```python
from build123d import *

# Parameters (mm, degrees)
F1_DEPTH = 25.4
F3_R     = 6.35
F4_DEPTH = 25.4
F6_DEPTH = 25.4
F7_W     = 12.7
F7_H     = 7.132675
F8_DEPTH = 19.05


with BuildPart() as f1:
    # F0 (on Front) → F1 (new body)
    with BuildSketch(Plane.XZ):
        Polygon((0, 44.45), (0, 0), (57.15, 0), (57.15, 12.7), (12.7, 12.7), (12.7, 44.45), align=None)
    extrude(amount=F1_DEPTH)

    # F3 (on face) → F4 (cut)
    with BuildSketch(Plane.XY.offset(12.7)):
        with Locations((26.631284, -12.7)):
            Circle(F3_R)
        with Locations((45.681284, -12.7)):
            Circle(F3_R)
    extrude(amount=-F4_DEPTH, mode=Mode.SUBTRACT)

    # F5 (on face) → F6 (cut)
    with BuildSketch(Plane.XY.offset(12.7)):
        with BuildLine():
            ThreePointArc((46.05227, 0), (56.65458, -12.572447), (46.362385, -25.4))
            Line((46.362385, -25.4), (57.15, -25.4))
            Line((57.15, -25.4), (57.15, 0))
            Line((57.15, 0), (46.05227, 0))
        make_face()
    extrude(amount=-F6_DEPTH, mode=Mode.SUBTRACT)

    # F7 (on face) → F8 (cut)
    with BuildSketch(Plane.XY.offset(44.45)):
        with Locations((6.35, -11.474303)):
            Rectangle(F7_W, F7_H)
    extrude(amount=-F8_DEPTH, mode=Mode.SUBTRACT)


solid = f1.part
```
Input: part model. Units: mm. Frame: model coordinates. A direction names the side the tool comes from. Round coordinates to 2 decimals unless told otherwise and drop trailing zeros. Loops run counter-clockwise (first coordinate to the right, second up) from the corner with the lowest first, then second, coordinate; pieces in that order, holes last. Notation, with made-up numbers: (65, 42.5) - (97, 42.5) arc R32 cw to (97, 79.5) - close; hole circle Ø2 at (8, 59). An arc over 180 degrees is marked (long way). One line per item, written item: value. Start each with the question number.
(1) Ray query, line 1 (X direction, y = -7, z = 8); line 2 (X direction, y = -13.75, z = 10.5); line 3 (Y direction, x = 48, z = 8). Return the intervals inside material, ascending. Write a range as [from, to].
(2) Draft query along X for faces 1 (the flat face through (0, -13, 23)), 2 (the cylindrical face through (51.55, -15.13, 6.44)), 3 (the flat face through (12.7, -13, 25)), 4 (the flat face through (6, -7.908, 35)). Return one class per face: +X half, -X half, draft (parallel to the pull), parting line (faces both ways), or undercut.
(3) Contact query for flat-ended pins moving along their axis: P1, Ø1.5, axis at x = 15, y = -6.5, coming from the +Z side; P2, Ø1.5, axis at y = -15.5, z = 28.5, coming from the +X side; P3, Ø3.5, axis at x = 5.5, y = -10, coming from the +Z side. Output: stop coordinate, or through.
(4) Access query for faces 5 (the flat face through (6, -11, 25.4)), 6 (the flat face through (35, -13, 12.7)), 7 (the flat face through (12.55, -25.4, 12.66)). Directions: +Z, -Z, +X, -X, +Y, -Y. A direction counts if a zero-diameter tool reaches every point of the face in a straight line with its end or side. Return the directions, or none.
(5) Section A-A, the plane z = 26.5. Return loops of the section in (x, y).
(6) Section C-C, the plane x = 51. Return loops of the section in (y, z), plus the area to 3 significant figures.
(7) Section D-D, the plane y = -12.7. Return loops of the section in (x, z), plus the area to 3 significant figures.
(8) Section B-B, the plane z = 11. Return loops of the section in (x, y), plus the area to 3 significant figures.
Results below:
1. line 1: [0, 23.83], [29.43, 42.88], [48.48, 55.32]
1. line 2: [0, 20.37], [32.89, 39.42], [51.94, 56.62]
1. line 3: [-24.94, -18.61], [-6.79, -0.52]
2. face 1: -X half
2. face 2: undercut
2. face 3: +X half
2. face 4: draft
3. P1: z = 12.7
3. P2: x = 12.7
3. P3: z = 25.4
4. face 5: +Z, +X, -X
4. face 6: +Z, +X, +Y, -Y
4. face 7: +Z, -Z, +X, -X, -Y
5. outline: (0, -25.4) - (12.7, -25.4) - (12.7, -15.04) - (0, -15.04) - close; (0, -7.91) - (12.7, -7.91) - (12.7, 0) - (0, 0) - close
6. outline: (-23.43, 0) - (-16.17, 0) - (-16.17, 12.7) - (-23.43, 12.7) - close; (-9.23, 0) - (-2.03, 0) - (-2.03, 12.7) - (-9.23, 12.7) - close
6. area: 184 mm^2
7. outline: (0, 0) - (20.28, 0) - (20.28, 12.7) - (12.7, 12.7) - (12.7, 25.4) - (0, 25.4) - close; (32.98, 0) - (39.33, 0) - (39.33, 12.7) - (32.98, 12.7) - close; (52.03, 0) - (56.66, 0) - (56.66, 12.7) - (52.03, 12.7) - close
7. area: 558 mm^2
8. outline: (0, -25.4) - (46.36, -25.4) arc R12.94 ccw to (46.05, 0) - (0, 0) - close; hole circle Ø12.7 at (26.63, -12.7); hole circle Ø12.7 at (45.68, -12.7)
8. area: 1,120 mm^2
